Verification items for the finished model (mm, model axes). Round coordinates to 2 decimals unless told otherwise and drop trailing zeros. Loops run counter-clockwise (first coordinate to the right, second up) from the corner with the lowest first, then second, coordinate; pieces in that order, holes last. Notation, with made-up numbers: (-29, 79.5) - (-6, 79.5) arc R28 ccw to (-6, 108.5) - close; hole circle Ø6 at (84, 62.5). An arc over 180 degrees is marked (long way). Use CSV: the item, a comma, the result in double quotes.
```python
from build123d import *

# Parameters (mm, degrees)
SKETCH1_W           = 30
SKETCH1_H           = 20
SKETCH1_W_2         = 2
SKETCH1_H_2         = 5
BOSS_EXTRUDE1_DEPTH = 2
SKETCH2_R           = 1.5
CUT_EXTRUDE1_DEPTH  = 10


with BuildPart() as part:
    # Sketch1 → Boss-Extrude1 (new body)
    with BuildSketch(Plane(origin=(0, 0, 0), x_dir=(1, 0, 0), z_dir=(0, 1, 0))):
        Rectangle(SKETCH1_W, SKETCH1_H)
        with Locations((-1, 5)):
            Rectangle(SKETCH1_W_2, SKETCH1_H_2, mode=Mode.SUBTRACT)
        with Locations((-1, -5)):
            Rectangle(SKETCH1_W_2, SKETCH1_H_2, mode=Mode.SUBTRACT)
    extrude(amount=BOSS_EXTRUDE1_DEPTH)

    # Sketch2 → Cut-Extrude1 (cut)
    with BuildSketch(Plane(origin=(0, 2, 0), x_dir=(1, 0, 0), z_dir=(0, 1, 0))):
        with Locations(Location((-10, 5, 0), (0, 0, 270))):
            Circle(SKETCH2_R)
        with Locations(Location((-10, -5, 0), (0, 0, 270))):
            Circle(SKETCH2_R)
    extrude(amount=-CUT_EXTRUDE1_DEPTH, mode=Mode.SUBTRACT)


solid = part.part
```
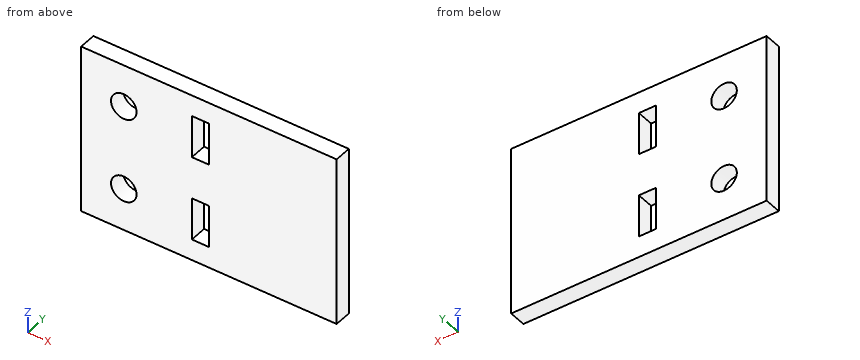
1) Cross-section at B-B, the plane x = -10. Record the cut outline in (y, z), then the cut area to 3 significant figures.
Returned:
outline,"(0, -10) - (2, -10) - (2, -6.5) - (0, -6.5) - close; (0, -3.5) - (2, -3.5) - (2, 3.5) - (0, 3.5) - close; (0, 6.5) - (2, 6.5) - (2, 10) - (0, 10) - close"
area,"28.0 mm²"
2) Thickness scan on probe 1 along X at (y, z) = (0.9, -5); probe 2 along X at (y, z) = (0.9, -6.25); probe 3 along X at (y, z) = (0.6, -6.75). Record the ranges inside material, lowest first. Write a range as [from, to].
Returned:
probe 1,"x = [-15, -11.5], [-8.5, -2], [0, 15]"
probe 2,"x = [-15, -10.83], [-9.17, -2], [0, 15]"
probe 3,"x = [-15, -2], [0, 15]"
3) Gauge pin test, flat end, axial feed: pin 1 Ø2.5 at (x, z) = (-10, -5) entering from +Y. Record the tip position at first contact, or that the pin passes through.
Returned:
pin 1,"passes through"
4) Cross-section at A-A, the plane z = -5. Record the cut outline in (x, y).
Returned:
outline,"(-15, 0) - (-11.5, 0) - (-11.5, 2) - (-15, 2) - close; (-8.5, 0) - (-2, 0) - (-2, 2) - (-8.5, 2) - close; (0, 0) - (15, 0) - (15, 2) - (0, 2) - close"
5) Cross-section at C-C, the plane y = 1.55. Record the cut outline in (x, z), then the cut area to 3 significant figures.
Returned:
outline,"(-15, -10) - (15, -10) - (15, 10) - (-15, 10) - close; hole circle Ø3 at (-10, -5); hole circle Ø3 at (-10, 5); hole (-2, -7.5) - (0, -7.5) - (0, -2.5) - (-2, -2.5) - close; hole (-2, 2.5) - (0, 2.5) - (0, 7.5) - (-2, 7.5) - close"
area,"566 mm²"
